Geometry check sheet. Reference: the model listing, model coordinates, mm. Face numbers are marked on the shaded views. A direction names the side the tool comes from. Give positions to 0.01 mm unless a question says otherwise; leave off trailing zeros. Write each loop counter-clockwise with the first axis right and the second up, starting at its lowest first coordinate (ties: lowest second). Pieces come first, ordered by that corner, then holes. Notation, with made-up numbers: (-19.75, 81) -> (6.25, 81) arc R6 ccw to (6.25, 89) -> close; hole circle Ø1 at (31.25, 69). An arc over 180 degrees is marked (long way). Write item = value, one per line. Start each with the question number.
1. Depth check by flat-ended pin: P1, Ø2, axis at x = 11, z = -13, coming from the +Y side; P2, Ø3, axis at y = -13.5, z = 14.5, coming from the +X side; P3, Ø6, axis at x = 12.02, z = -12.02, coming from the -Y side; P4, Ø3.5, axis at x = -12.02, z = -12.02, coming from the +Y side. Enter the tip coordinate at first touch or a pass-through.
2. Cross-section at A-A, the plane x = 0. Record the cut outline in (y, z).
3. Cross-section at C-C, the plane x = 39.5. Record the cut outline in (y, z), plus the area to 3 significant figures.
4. Thickness scan on line 1 along X through (y, z) = (-16.5, -12.5); line 2 along Y through (x, z) = (19, -15); line 3 along Y through (x, z) = (49.5, 20). Record the ranges inside material, lowest first.
5. Set-up check for the marked faces 4, 5 and 6: record each of +Z, -Z, +X, -X, +Y, -Y from which the full face is reachable in a straight line by a thin tool's end or side.
6. Cross-section at D-D, the plane z = 0. Record the cut outline in (x, y).
7. Mould release check, pull along X, two halves, no side actions. Record for the marked faces 1, 2 and 3: pulls with the +X half, pulls with the -X half, needs draft (parallel to the pull), parting line crosses it, or undercut.
8. Cross-section at B-B, the plane z = 8.5. Record the cut outline in (x, y), plus the area to 3 significant figures.
```python
from build123d import *

# Parameters (mm, degrees)
SKETCH1_W          = 44
SKETCH1_H          = 46
SKETCH1_R          = 12.5
SKETCH1_R_2        = 2.25
BASE_FLANGE1_DEPTH = 2
EDGE_FLANGE1_DEPTH = 46
EDGE_FLANGE2_DEPTH = 46
CUT_EXTRUDE1_DEPTH = 2
FILLET1_R          = 4


# Sheet-metal steps are written as plain solids
with BuildPart() as part:
    # Sketch1 → Base-Flange1 (new body)
    with BuildSketch(Plane(origin=(0, 0, 0), x_dir=(1, 0, 0), z_dir=(0, 1, 0))):
        Rectangle(SKETCH1_W, SKETCH1_H)
        with Locations(Location((0, 0, 0), (0, 0, 270))):
            Circle(SKETCH1_R, mode=Mode.SUBTRACT)
        with Locations(Location((12.02081528, 12.02081528, 0), (0, 0, 270))):
            Circle(SKETCH1_R_2, mode=Mode.SUBTRACT)
        with Locations(Location((12.02081528, -12.02081528, 0), (0, 0, 270))):
            Circle(SKETCH1_R_2, mode=Mode.SUBTRACT)
        with Locations(Location((-12.02081528, -12.02081528, 0), (0, 0, 270))):
            Circle(SKETCH1_R_2, mode=Mode.SUBTRACT)
        with Locations(Location((-12.02081528, 12.02081528, 0), (0, 0, 270))):
            Circle(SKETCH1_R_2, mode=Mode.SUBTRACT)
    extrude(amount=-BASE_FLANGE1_DEPTH)

    # Edge-Flange1 section (across the edge) → Edge-Flange1 (add)
    with BuildSketch(Plane(origin=(23.2, -2, -23), x_dir=(-1, 0, 0), z_dir=(0, 0, 1))):
        with BuildLine():
            Line((-2, 1.2), (-2, 25))
            Line((-2, 25), (0, 25))
            Line((0, 25), (0, 1.2))
            ThreePointArc((0, 1.2), (0.351471863, 0.351471863), (1.2, 0))
            Line((1.2, 0), (1.2, -2))
            ThreePointArc((1.2, -2), (-1.0627417, -1.0627417), (-2, 1.2))
        make_face()
    extrude(amount=EDGE_FLANGE1_DEPTH)

    # Edge-Flange2 section (across the edge) → Edge-Flange2 (add)
    with BuildSketch(Plane(origin=(25.2, -28.2, 23), x_dir=(0, 1, 0), z_dir=(0, 0, -1))):
        with BuildLine():
            Line((-2, 1.2), (-2, 28))
            Line((-2, 28), (0, 28))
            Line((0, 28), (0, 1.2))
            ThreePointArc((0, 1.2), (0.351471863, 0.351471863), (1.2, 0))
            Line((1.2, 0), (1.2, -2))
            ThreePointArc((1.2, -2), (-1.0627417, -1.0627417), (-2, 1.2))
        make_face()
    extrude(amount=EDGE_FLANGE2_DEPTH)

    # Sketch12 → Cut-Extrude1 (cut)
    with BuildSketch(Plane(origin=(0, -28.2, 0), x_dir=(1, 0, 0), z_dir=(0, 1, 0))):
        with BuildLine():
            Line((38.561884659, 16.5), (41.061884659, 16.5))
            ThreePointArc((41.061884659, 16.5), (43.561884659, 14), (41.061884659, 11.5))
            Line((41.061884659, 11.5), (38.561884659, 11.5))
            ThreePointArc((38.561884659, 11.5), (36.061884659, 14), (38.561884659, 16.5))
        make_face()
        with BuildLine():
            Line((38.561884659, -16.5), (41.061884659, -16.5))
            ThreePointArc((41.061884659, -16.5), (43.561884659, -14), (41.061884659, -11.5))
            Line((41.061884659, -11.5), (38.561884659, -11.5))
            ThreePointArc((38.561884659, -11.5), (36.061884659, -14), (38.561884659, -16.5))
        make_face()
    extrude(amount=-CUT_EXTRUDE1_DEPTH, mode=Mode.SUBTRACT)

    # Fillet1
    fillet1_edges = [part.edges().sort_by_distance(p)[0] for p in [
        (53.2, -29.2, 23),
        (53.2, -29.2, -23),
        (-22, -1, 23),
        (-22, -1, -23),
    ]]
    fillet(fillet1_edges, radius=FILLET1_R)


solid = part.part
```
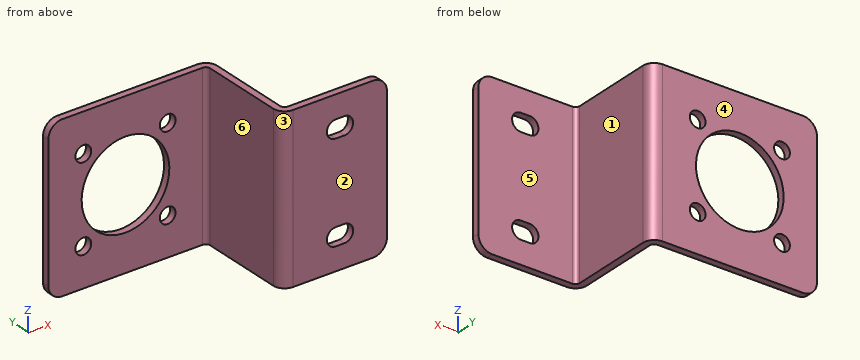
Answers:
q1.P1 = 0
q1.P2 = 25.2
q1.P3 = -2
q1.P4 = through
q2.outline = (-2, -23) -> (0, -23) -> (0, -12.5) -> (-2, -12.5) -> close; (-2, 12.5) -> (0, 12.5) -> (0, 23) -> (-2, 23) -> close
q3.outline = (-30.2, -23) -> (-28.2, -23) -> (-28.2, -16.5) -> (-30.2, -16.5) -> close; (-30.2, -11.5) -> (-28.2, -11.5) -> (-28.2, 11.5) -> (-30.2, 11.5) -> close; (-30.2, 16.5) -> (-28.2, 16.5) -> (-28.2, 23) -> (-30.2, 23) -> close
q3.area = 72.0 mm^2
q4.line_1 = 23.2 to 25.2
q4.line_2 = -2 to 0
q4.line_3 = -30.2 to -28.2
q5.face_4 = +Z, -Z, +X, -X, +Y
q5.face_5 = +Z, -Z, +X, +Y
q5.face_6 = +Z, -Z, -X, -Y
q6.outline = (-22, -2) -> (-12.5, -2) -> (-12.5, 0) -> (-22, 0) -> close; (12.5, -2) -> (22, -2) arc R1.2 cw to (23.2, -3.2) -> (23.2, -27) arc R3.2 ccw to (26.4, -30.2) -> (53.2, -30.2) -> (53.2, -28.2) -> (26.4, -28.2) arc R1.2 cw to (25.2, -27) -> (25.2, -3.2) arc R3.2 ccw to (22, 0) -> (12.5, 0) -> close
q7.face_1 = pulls with the +X half
q7.face_2 = needs draft
q7.face_3 = pulls with the -X half
q8.outline = (-22, -2) -> (-9.17, -2) -> (-9.17, 0) -> (-22, 0) -> close; (9.17, -2) -> (22, -2) arc R1.2 cw to (23.2, -3.2) -> (23.2, -27) arc R3.2 ccw to (26.4, -30.2) -> (53.2, -30.2) -> (53.2, -28.2) -> (26.4, -28.2) arc R1.2 cw to (25.2, -27) -> (25.2, -3.2) arc R3.2 ccw to (22, 0) -> (9.17, 0) -> close
q8.area = 166 mm^2
